Geometry check sheet. Reference: the model listing, model coordinates, mm. Face numbers are marked on the shaded views. A direction names the side the tool comes from. Give positions to 0.01 mm unless a question says otherwise; leave off trailing zeros. Loops run counter-clockwise (first coordinate to the right, second up) from the corner with the lowest first, then second, coordinate; pieces in that order, holes last.
1. Go/stop test with flat-tipped pins: pin 1 Ø1.5 at (x, z) = (-1, 0) entering from +Y; pin 2 Ø3 at (y, z) = (7.5, -1) entering from +X; pin 3 Ø4 at (x, y) = (-1, 5.5) entering from +Z. Record where each tip stops, or that it passes through.
2. Tool access check on the marked faces 4, 5, 6 and 7. Record the directions out of +Z, -Z, +X, -X, +Y, -Y that give a thin tool (end or side, any length) a straight path to the whole face; none if there is none.
3. Cross-section at C-C, the plane z = 0.4. Record the cut outline in (x, y).
4. Cross-section at A-A, the plane x = 4. Record the cut outline in (y, z).
5. Release check for a two-part mould opening along Z. For the marked faces 1, 2 and 3 record: +Z half, -Z half, draft (parallel to the pull), parting line (faces both ways), or undercut.
6. Material ranges on L1, parallel to Y at x = 0.5, z = 1.7; L2, parallel to Z at x = -2.5, y = 3.75; L3, parallel to X at y = 2.25, z = -0.8, recorded low to high.
7. Cross-section at B-B, the plane z = 2.05. Record the cut outline in (x, y).
8. Cross-section at D-D, the plane x = 3. Record the cut outline in (y, z).
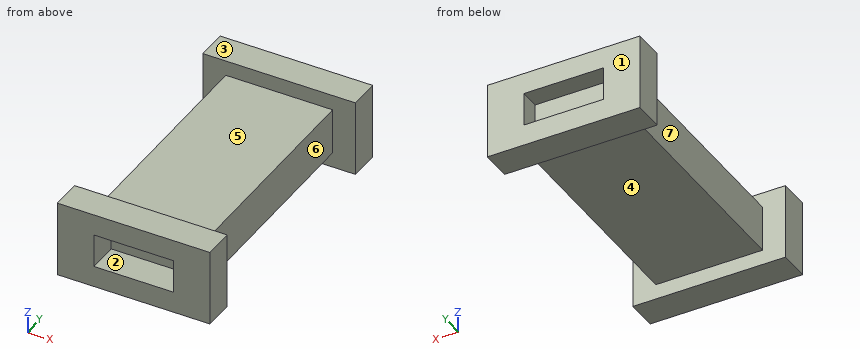
Autodesk Inventor part; units mm, degrees
ref_plane "YZ Plane" through (0, 0, 0) normal (1, 0, 0) x (0, 1, 0)
ref_plane "XZ Plane" through (0, 0, 0) normal (0, 1, 0) x (-1, 0, 0)
ref_plane "XY Plane" through (0, 0, 0) normal (0, 0, 1) x (1, 0, 0)
sketch "草圖7" plane through (0, 0, 0) normal (0, 1, 0) x (-1, 0, 0)
  line L0 (5, 2.5) -> (-5, 2.5)
  line L1 (-5, 2.5) -> (-5, -2.5)
  line L2 (-5, -2.5) -> (5, -2.5)
  line L3 (5, -2.5) -> (5, 2.5)
  line L4 (5, 2.5) -> (-5, -2.5) construction
  line L5 (-5, 2.5) -> (5, -2.5) construction
  line L6 (2.6, 1.1) -> (-2.6, 1.1)
  line L7 (-2.6, 1.1) -> (-2.6, -1.1)
  line L8 (-2.6, -1.1) -> (2.6, -1.1)
  line L9 (2.6, -1.1) -> (2.6, 1.1)
  line L10 (2.6, 1.1) -> (-2.6, -1.1) construction
  line L11 (-2.6, 1.1) -> (2.6, -1.1) construction
  point P0 (0, 0)
  dimension "d18" = 10
  dimension "d19" = 5
  dimension "d20" = 2.2
  dimension "d21" = 5.2
extrude "擠出7" add sketch "草圖7" against normal blind 2
sketch "草圖8" plane through (0, 0, 0) normal (0, 1, 0) x (1, 0, 0)
  line L0 (-3.5, -1.5) -> (3.5, -1.5)
  line L1 (3.5, -1.5) -> (3.5, 1.5)
  line L2 (3.5, 1.5) -> (-3.5, 1.5)
  line L3 (-3.5, 1.5) -> (-3.5, -1.5)
  line L4 (-3.5, -1.5) -> (3.5, 1.5) construction
  line L5 (3.5, -1.5) -> (-3.5, 1.5) construction
  point P0 (0, 0)
  dimension "d24" = 7
  dimension "d25" = 3
extrude "擠出8" add sketch "草圖8" along normal blind 15
sketch "草圖9" plane through (0, 15, 0) normal (0, 1, 0) x (1, 0, 0)
  line L0 (5, -2.5) -> (5, 2.5)
  line L1 (-5, -2.5) -> (5, -2.5)
  line L2 (5, -2.5) -> (5, 2.5)
  line L3 (5, 2.5) -> (-5, 2.5)
  line L4 (-5, 2.5) -> (-5, -2.5)
  line L5 (-5, -2.5) -> (5, 2.5) construction
  line L6 (5, -2.5) -> (-5, 2.5) construction
  point P0 (0, 0)
extrude "擠出9" add sketch "草圖9" along normal blind 2
sketch "草圖10" plane through (0, 17, 0) normal (0, 1, 0) x (1, 0, 0)
  line L0 (-2.6, 1.1) -> (2.6, 1.1)
  line L1 (-2.6, -1.1) -> (2.6, -1.1)
  line L2 (2.6, -1.1) -> (2.6, 1.1)
  line L3 (2.6, 1.1) -> (-2.6, 1.1)
  line L4 (-2.6, 1.1) -> (-2.6, -1.1)
  line L5 (-2.6, -1.1) -> (2.6, 1.1) construction
  line L6 (2.6, -1.1) -> (-2.6, 1.1) construction
  point P0 (0, 0)
extrude "擠出10" cut sketch "草圖10" against normal blind 1.3
properties part number "差分線圈感應"
Result:
1. pin 1: stops at y = 15.7
1. pin 2: stops at x = 3.5
1. pin 3: stops at z = 1.5
2. face 4: -Z, +X, -X
2. face 5: +Z, +X, -X
2. face 6: +Z, -Z, +X
2. face 7: +Z, -Z, -X
3. outline: (-5, -2) - (-2.6, -2) - (-2.6, 0) - (2.6, 0) - (2.6, -2) - (5, -2) - (5, 0) - (3.5, 0) - (3.5, 15) - (5, 15) - (5, 17) - (2.6, 17) - (2.6, 15.7) - (-2.6, 15.7) - (-2.6, 17) - (-5, 17) - (-5, 15) - (-3.5, 15) - (-3.5, 0) - (-5, 0) - close
4. outline: (-2, -2.5) - (0, -2.5) - (0, 2.5) - (-2, 2.5) - close; (15, -2.5) - (17, -2.5) - (17, 2.5) - (15, 2.5) - close
5. face 1: draft
5. face 2: undercut
5. face 3: +Z half
6. L1: y = -2 to 0, 15 to 17
6. L2: z = -1.5 to 1.5
6. L3: x = -3.5 to 3.5
7. outline: (-5, -2) - (5, -2) - (5, 0) - (-5, 0) - close; (-5, 15) - (5, 15) - (5, 17) - (-5, 17) - close
8. outline: (-2, -2.5) - (0, -2.5) - (0, -1.5) - (15, -1.5) - (15, -2.5) - (17, -2.5) - (17, 2.5) - (15, 2.5) - (15, 1.5) - (0, 1.5) - (0, 2.5) - (-2, 2.5) - close
